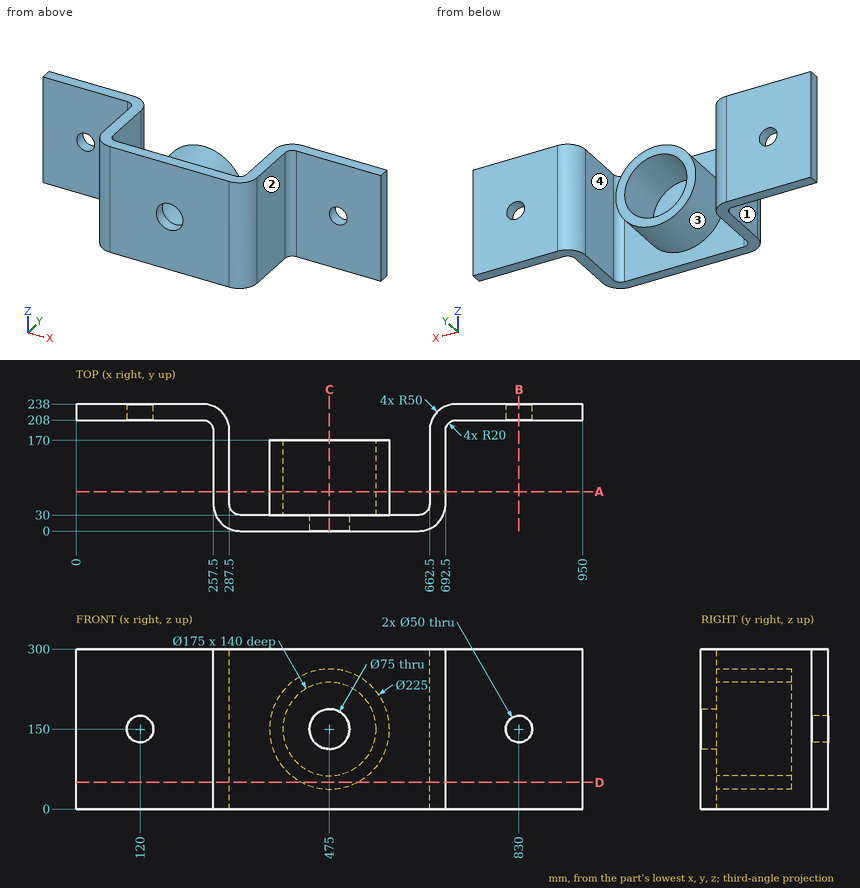
Can you work these out from the drawing? Everything is in mm from the part's minimum corner. A direction names the side the tool comes from. Coordinates: 2 decimals unless noted, no trailing zeros. Loops run counter-clockwise (first coordinate to the right, second up) from the corner with the lowest first, then second, coordinate; pieces in that order, holes last.
1. Imagine slicing it at C-C, the plane x = 475. Please give me the cut outline in (y, z), and give its area (4 significant figures).
2. Imagine slicing it at D-D, the plane z = 50. Please give me the cut outline in (x, y), and give its area (3 significant figures).
3. For P1, Ø5, axis at y = 112, z = 232.5, coming from the -X side; P2, Ø1, axis at y = 209, z = 102.5, coming from the -X side; P3, Ø6, axis at x = 223.5, z = 71, coming from the -Y side, each with a flat end and sliding along its axis, tell me the tip position at first contact or that it passes through.
4. I need wall thicknesses on L1, parallel to X at y = 126.5, z = 145; L2, parallel to Z at x = 120, y = 222; L3, parallel to X at y = 76.5, z = 150. Which ranges of each line are inside material? Lowest first, please.
5. Imagine slicing it at B-B, the plane x = 830. Please give me the cut outline in (y, z).
6. Imagine slicing it at A-A, the plane y = 74. Please give me the cut outline in (x, z), and give its area (3 significant figures).
7. For the marked faces 1, 2, 3 and 4, which set-ups out of +Z, -Z, +X, -X, +Y, -Y let a thin tool reach every point of the face, with its end or its side?
Taken from the geometry:
1. outline: (0, 0) - (30, 0) - (30, 37.5) - (170, 37.5) - (170, 62.5) - (30, 62.5) - (30, 112.5) - (0, 112.5) - close; (0, 187.5) - (30, 187.5) - (30, 237.5) - (170, 237.5) - (170, 262.5) - (30, 262.5) - (30, 300) - (0, 300) - close
1. area: 13,750 mm2
2. outline: (0, 208) - (237.5, 208) arc R20 cw to (257.5, 188) - (257.5, 50) arc R50 ccw to (307.5, 0) - (642.5, 0) arc R50 ccw to (692.5, 50) - (692.5, 188) arc R20 cw to (712.5, 208) - (950, 208) - (950, 238) - (712.5, 238) arc R50 ccw to (662.5, 188) - (662.5, 50) arc R20 cw to (642.5, 30) - (526.54, 30) - (526.54, 170) - (423.46, 170) - (423.46, 30) - (307.5, 30) arc R20 cw to (287.5, 50) - (287.5, 188) arc R50 ccw to (237.5, 238) - (0, 238) - close
2. area: 53,600 mm2
3. P1: stops at x = 257.5
3. P2: stops at x = 0
3. P3: stops at y = 208
4. L1: x = 257.5 to 287.5, 362.61 to 387.64, 562.36 to 587.39, 662.5 to 692.5
4. L2: z = 0 to 125, 175 to 300
4. L3: x = 257.5 to 287.5, 362.5 to 387.5, 562.5 to 587.5, 662.5 to 692.5
5. outline: (208, 0) - (238, 0) - (238, 125) - (208, 125) - close; (208, 175) - (238, 175) - (238, 300) - (208, 300) - close
6. outline: (257.5, 0) - (287.5, 0) - (287.5, 300) - (257.5, 300) - close; circle Ø225 at (475, 150); (662.5, 0) - (692.5, 0) - (692.5, 300) - (662.5, 300) - close; hole circle Ø175 at (475, 150)
6. area: 33,700 mm2
7. face 1: +Z, -Z, -X, -Y
7. face 2: +Z, -Z, +X, -Y
7. face 3: +Y
7. face 4: +Z, -Z, +Y
